```python
from build123d import *

# Parameters (mm, degrees)
SKETCH1_R               = 5
BOSS_EXTRUDE1_DEPTH     = 33
SKETCH2_R               = 8
BOSS_EXTRUDE2_DEPTH     = 95
CUT_EXTRUDE1_START      = -8
SKETCH3_OUTSIDE_W       = 43.996
SKETCH3_OUTSIDE_H       = 43.996
SKETCH3_OUTSIDE_R       = 7.6
CUT_EXTRUDE1_DEPTH      = 1.1
CUT_EXTRUDE2_START      = -25.1
SKETCH3_2_OUTSIDE_W     = 43.996
SKETCH3_2_OUTSIDE_H     = 43.996
SKETCH3_2_OUTSIDE_R     = 7.6
CUT_EXTRUDE2_DEPTH      = 1.1
CUT_EXTRUDE3_START      = 16
SKETCH4_OUTSIDE_W       = 43.996
SKETCH4_OUTSIDE_H       = 43.996
SKETCH4_OUTSIDE_R       = 4.8
CUT_EXTRUDE3_DEPTH      = 1.1
SKETCH5_R               = 2.1
CUT_EXTRUDE4_DEPTH      = 10
CUT_EXTRUDE5_START      = -15
CUT_EXTRUDE5_DEPTH      = 15
FILLET1_R               = 2
CUT_EXTRUDE6_DEPTH      = 129.499027333
CUT_EXTRUDE6_DEPTH_BACK = 40
FILLET2_R               = 2.5
CHAMFER1_SIZE           = 0.5


with BuildPart() as part:
    # Sketch1 → Boss-Extrude1 (new body)
    with BuildSketch(Plane(origin=(0, 0, 0), x_dir=(1, 0, 0), z_dir=(0, 1, 0))):
        with Locations(Location((0, 0, 0), (0, 0, 270))):
            Circle(SKETCH1_R)
    extrude(amount=BOSS_EXTRUDE1_DEPTH)

    # Sketch2 → Boss-Extrude2 (add)
    with BuildSketch(Plane.XZ):
        with Locations(Location((0, 0, 0), (0, 0, 270))):
            Circle(SKETCH2_R)
    extrude(amount=BOSS_EXTRUDE2_DEPTH)

    # Sketch3 outside → Cut-Extrude1 (cut)
    with BuildSketch(Plane(origin=(0, 0, 0), x_dir=(1, 0, 0), z_dir=(0, 1, 0)).offset(CUT_EXTRUDE1_START)):
        Rectangle(SKETCH3_OUTSIDE_W, SKETCH3_OUTSIDE_H)
        with Locations(Location((0, 0, 0), (0, 0, 270))):
            Circle(SKETCH3_OUTSIDE_R, mode=Mode.SUBTRACT)
    extrude(amount=-CUT_EXTRUDE1_DEPTH, mode=Mode.SUBTRACT)

    # Sketch3<2> outside → Cut-Extrude2 (cut)
    with BuildSketch(Plane(origin=(0, 0, 0), x_dir=(1, 0, 0), z_dir=(0, 1, 0)).offset(CUT_EXTRUDE2_START)):
        Rectangle(SKETCH3_2_OUTSIDE_W, SKETCH3_2_OUTSIDE_H)
        with Locations(Location((0, 0, 0), (0, 0, 270))):
            Circle(SKETCH3_2_OUTSIDE_R, mode=Mode.SUBTRACT)
    extrude(amount=-CUT_EXTRUDE2_DEPTH, mode=Mode.SUBTRACT)

    # Sketch4 outside → Cut-Extrude3 (cut)
    with BuildSketch(Plane(origin=(0, 0, 0), x_dir=(1, 0, 0), z_dir=(0, 1, 0)).offset(CUT_EXTRUDE3_START)):
        Rectangle(SKETCH4_OUTSIDE_W, SKETCH4_OUTSIDE_H)
        with Locations(Location((0, 0, 0), (0, 0, 270))):
            Circle(SKETCH4_OUTSIDE_R, mode=Mode.SUBTRACT)
    extrude(amount=CUT_EXTRUDE3_DEPTH, mode=Mode.SUBTRACT)

    # Sketch5 → Cut-Extrude4 (cut)
    with BuildSketch(Plane.XZ.offset(95)):
        with Locations(Location((0, 0, 0), (0, 0, 270))):
            Circle(SKETCH5_R)
    extrude(amount=-CUT_EXTRUDE4_DEPTH, mode=Mode.SUBTRACT)

    # Sketch6 → Cut-Extrude5 (cut)
    with BuildSketch(Plane(origin=(0, 33, 0), x_dir=(1, 0, 0), z_dir=(0, 1, 0)).offset(CUT_EXTRUDE5_START)):
        with BuildLine():
            Line((4.582575695, 2), (2.5, 2))
            Line((2.5, 2), (2.5, -2))
            Line((2.5, -2), (4.582575695, -2))
            ThreePointArc((4.582575695, -2), (5, 0), (4.582575695, 2))
        make_face()
    extrude(amount=CUT_EXTRUDE5_DEPTH, mode=Mode.SUBTRACT)

    # Fillet1
    fillet1_edges = [part.edges().sort_by_distance(p)[0] for p in [
        (3.541287847, 18, 2),
        (3.541287847, 18, -2),
    ]]
    fillet(fillet1_edges, radius=FILLET1_R - 0.0001)  # a hair under: the kernel refuses the full size

    # Sketch7 → Cut-Extrude6 (cut, two sides: drawn at the far end of the back side and taken through both)
    with BuildSketch(Plane.XZ.offset(95).offset(-CUT_EXTRUDE6_DEPTH_BACK)):
        Polygon((55.20729194, 2.5), (7.599342077, 2.5), (5, 2.5), (5, -2.5), (7.599342077, -2.5), (55.20729194, -2.5), (150.423191666, -2.5), (150.423191666, 2.5), align=None)
    extrude(amount=CUT_EXTRUDE6_DEPTH + CUT_EXTRUDE6_DEPTH_BACK, mode=Mode.SUBTRACT)

    # Fillet2
    fillet2_edges = [part.edges().sort_by_distance(p)[0] for p in [
        (6.299671038, -55, 2.5),
        (6.299671038, -55, -2.5),
    ]]
    fillet(fillet2_edges, radius=FILLET2_R - 0.0001)  # a hair under: the kernel refuses the full size

    # Chamfer1
    chamfer1_edges = [part.edges().sort_by_distance(p)[0] for p in [
        (0, 0, -5),
    ]]
    chamfer(chamfer1_edges, length=CHAMFER1_SIZE)


solid = part.part
```
Source: CAD feature listing. Evaluate the final solid. Frame: model axes, mm. A direction names the side the tool comes from. Give positions to 0.01 mm unless a question says otherwise; leave off trailing zeros. Loops run counter-clockwise (first coordinate to the right, second up) from the corner with the lowest first, then second, coordinate; pieces in that order, holes last. Notation, with made-up numbers: (87, 24) -> (128, 24) arc R30 cw to (128, 56) -> close; hole circle Ø1 at (22.25, 25). An arc over 180 degrees is marked (long way). Put each result on its own line as item: value. Start each with the question number.
1) Draft query along Y for faces 4 (the face through (-2.91, -8.54, 7.02)), 5 (the face through (2.5, 25, 0)), 6 (the face through (5.4, 0, -1.7)). Return one class per face: released by +Y, released by -Y, zero draft, split by the parting line, or undercut.
2) Cut plane A-A (y = -83). Return loops of the section in (x, z).
3) Material intervals for probe 1 along Y at (x, z) = (-6.25, -4.75); probe 2 along X at (y, z) = (-87.5, 0); probe 3 along Y at (x, z) = (1.25, 6.5), sorted ascending.
4) Contact query for flat-ended pins moving along their axis: P1, Ø2.5, axis at x = 0, z = 0, coming from the -Y side; P2, Ø1, axis at x = 3.5, y = 29.5, coming from the +Z side; P3, Ø3, axis at x = -4.5, y = -30.5, coming from the -Z side; P4, Ø1.5, axis at x = 0.5, y = -81, coming from the -Z side. Output: stop coordinate, or through.
5) Reachability of faces 1 (the face through (7, -56, -2)), 2 (the face through (-4.88, 24.94, -1.08)), 3 (the face through (4, 26, 2)) from +Z, -Z, +X, -X, +Y, -Y: full face, straight path, thin tool, end or side. Return the list, or none.
6) Cut plane B-B (y = 5.5). Return loops of the section in (x, z).
Results are:
1. face 4: undercut
1. face 5: zero draft
1. face 6: released by +Y
2. outline: (5, -2.5) -> (5, 2.5) -> (7.6, 2.5) arc R8 ccw (long way) to (7.6, -2.5) -> close
3. probe 1: y = -95 to -26.2, -25.1 to -9.1, -8 to 0
3. probe 2: x = -8 to -2.1, 2.1 to 5
3. probe 3: y = -95 to 0
4. P1: stops at y = -85
4. P2: stops at z = 4
4. P3: stops at z = -7.42
4. P4: stops at z = -8
5. face 1: +X, -Y
5. face 2: +Y
5. face 3: +X, +Y
6. outline: circle Ø10 at (0, 0)
